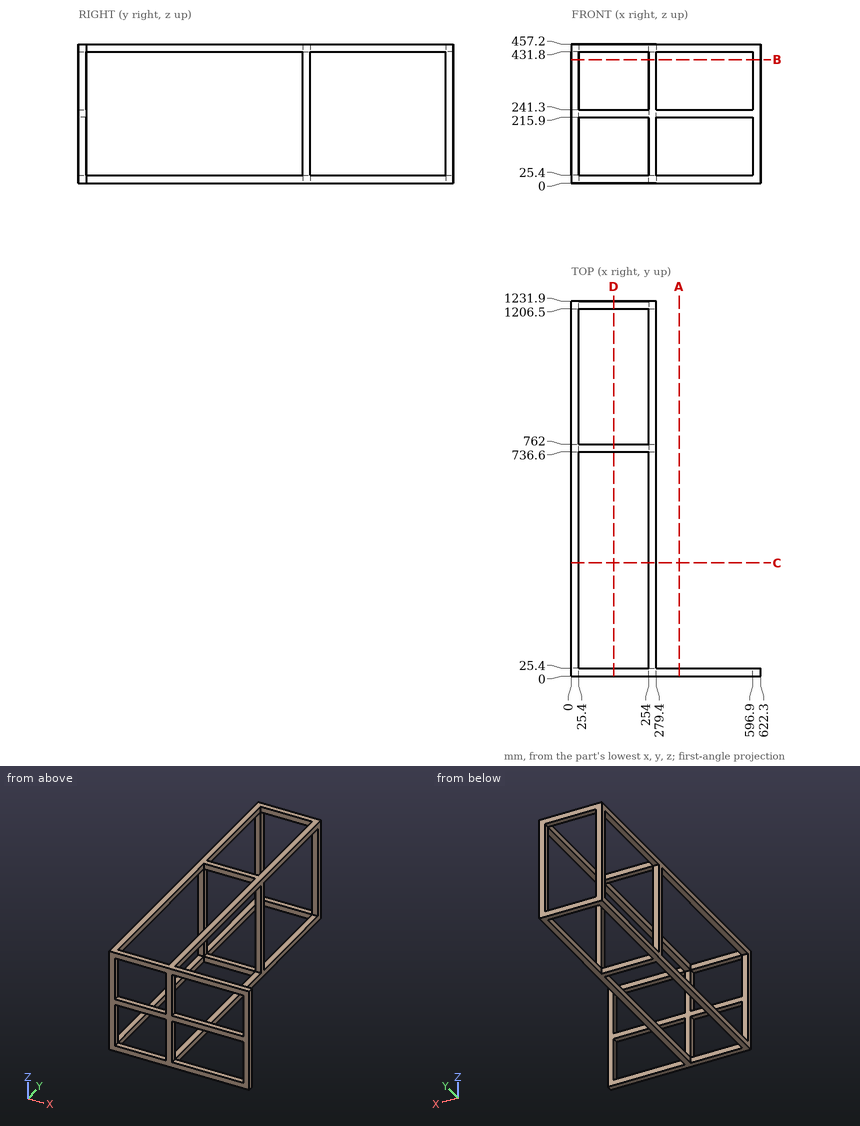
Design review of the part shown in the three views and the two pictorial views. Dimensions are in mm from the part's minimum x, y and z. Round coordinates to 2 decimals unless told otherwise and drop trailing zeros. Loops run counter-clockwise (first coordinate to the right, second up) from the corner with the lowest first, then second, coordinate; pieces in that order, holes last. Notation, with made-up numbers: (33, 13.25) -> (43, 13.25) arc R21 cw to (43, 34.25) -> close; hole circle Ø11 at (17.25, -31). An arc over 180 degrees is marked (long way). Answer as a JSON object with one key per item and string values. Group by question number.
1) We need section A-A on x = 354.5. Write out the cut boundary in (y, z).
2) We need section B-B on z = 406. Write out the cut boundary in (x, y).
3) For line 1 (X direction, y = 972, z = 432); line 2 (Z direction, x = 25, y = 109); line 3 (Y direction, x = 574.5, z = 433.5), list the stretches that pass through material, from the lowest coordinate up. Write a range as [from, to].
4) We need section C-C on y = 371.5. Write out the cut boundary in (x, z).
5) For pin 1 Ø7.5 at (y, z) = (1037.5, 16.5) entering from -X; pin 2 Ø12.5 at (y, z) = (925.5, 448) entering from +X, all flat-tipped, find the tip position at first contact; note any pin that passes through.
6) We need section D-D on x = 139. Write out the cut boundary in (y, z).
Result set:
{
 "1": {"outline": "(0, 0) -> (25.4, 0) -> (25.4, 25.4) -> (0, 25.4) -> close; (0, 215.9) -> (25.4, 215.9) -> (25.4, 241.3) -> (0, 241.3) -> close; (0, 431.8) -> (25.4, 431.8) -> (25.4, 457.2) -> (0, 457.2) -> close"},
 "2": {"outline": "(0, 0) -> (25.4, 0) -> (25.4, 25.4) -> (0, 25.4) -> close; (0, 736.6) -> (25.4, 736.6) -> (25.4, 762) -> (0, 762) -> close; (0, 1206.5) -> (25.4, 1206.5) -> (25.4, 1231.9) -> (0, 1231.9) -> close; (254, 0) -> (279.4, 0) -> (279.4, 25.4) -> (254, 25.4) -> close; (254, 736.6) -> (279.4, 736.6) -> (279.4, 762) -> (254, 762) -> close; (254, 1206.5) -> (279.4, 1206.5) -> (279.4, 1231.9) -> (254, 1231.9) -> close; (596.9, 0) -> (622.3, 0) -> (622.3, 25.4) -> (596.9, 25.4) -> close"},
 "3": {"line 1": "[0, 25.4], [254, 279.4]", "line 2": "[0, 25.4], [431.8, 457.2]", "line 3": "[0, 25.4]"},
 "4": {"outline": "(0, 0) -> (25.4, 0) -> (25.4, 25.4) -> (0, 25.4) -> close; (0, 431.8) -> (25.4, 431.8) -> (25.4, 457.2) -> (0, 457.2) -> close; (254, 0) -> (279.4, 0) -> (279.4, 25.4) -> (254, 25.4) -> close; (254, 431.8) -> (279.4, 431.8) -> (279.4, 457.2) -> (254, 457.2) -> close"},
 "5": {"pin 1": "x = 0", "pin 2": "x = 279.4"},
 "6": {"outline": "(0, 0) -> (25.4, 0) -> (25.4, 25.4) -> (0, 25.4) -> close; (0, 215.9) -> (25.4, 215.9) -> (25.4, 241.3) -> (0, 241.3) -> close; (0, 431.8) -> (25.4, 431.8) -> (25.4, 457.2) -> (0, 457.2) -> close; (736.6, 0) -> (762, 0) -> (762, 25.4) -> (736.6, 25.4) -> close; (736.6, 431.8) -> (762, 431.8) -> (762, 457.2) -> (736.6, 457.2) -> close; (1206.5, 0) -> (1231.9, 0) -> (1231.9, 25.4) -> (1206.5, 25.4) -> close; (1206.5, 431.8) -> (1231.9, 431.8) -> (1231.9, 457.2) -> (1206.5, 457.2) -> close"}
}
